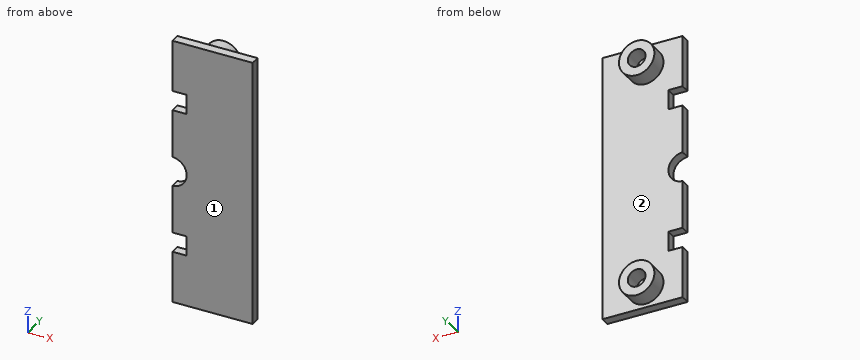
```python
from build123d import *

# Parameters (mm, degrees)
SKETCH1_W                       = 11.3
SKETCH1_H                       = 38
BASE_DEPTH                      = 1.3
SKETCH3_W                       = 2
SKETCH3_H                       = 2.8
SQUARE_NOTCH_DEPTH              = 20.864855902
SKETCH2_R                       = 2.1025
CIRCLE_DEPTH                    = 20.864855902
SKETCH4_R                       = 2.5
SKETCH4_R_2                     = 1.25
BOSSED_CYLINDER_WITH_HOLE_DEPTH = 2.4


with BuildPart() as part:
    # Sketch1 → BASE (new body)
    with BuildSketch(Plane(origin=(0, 0, 0), x_dir=(1, 0, 0), z_dir=(0, 1, 0))):
        Rectangle(SKETCH1_W, SKETCH1_H)
    extrude(amount=BASE_DEPTH)

    # Sketch3 → SQUARE NOTCH (cut, through all)
    with BuildSketch(Plane(origin=(0, 1.3, 0), x_dir=(1, 0, 0), z_dir=(0, 1, 0))):
        with Locations((-4.65, 10.3)):
            Rectangle(SKETCH3_W, SKETCH3_H)
    square_notch = extrude(amount=-SQUARE_NOTCH_DEPTH, mode=Mode.SUBTRACT)

    # SN Mirror1: SQUARE NOTCH across plane
    add(square_notch.mirror(Plane.XY), mode=Mode.SUBTRACT)

    # Sketch2 → CIRCLE (cut, through all)
    with BuildSketch(Plane(origin=(0, 1.3, 0), x_dir=(1, 0, 0), z_dir=(0, 1, 0))):
        with Locations((-5.7525, 0)):
            Circle(SKETCH2_R)
    extrude(amount=-CIRCLE_DEPTH, mode=Mode.SUBTRACT)

    # Sketch4 → BOSSED CYLINDER WITH HOLE (add)
    with BuildSketch(Plane(origin=(0, 1.3, 0), x_dir=(1, 0, 0), z_dir=(0, 1, 0))):
        with Locations(Location((-0.45, 16, 0), (0, 0, 270))):
            Circle(SKETCH4_R)
        with Locations(Location((-0.45, 16, 0), (0, 0, 270))):
            Circle(SKETCH4_R_2, mode=Mode.SUBTRACT)
    bossed_cylinder_with_hole = extrude(amount=BOSSED_CYLINDER_WITH_HOLE_DEPTH)

    # BCH Mirror2: BOSSED CYLINDER WITH HOLE across plane
    add(bossed_cylinder_with_hole.mirror(Plane.XY))


solid = part.part
```
The model under review builds one solid part; all positions refer to its coordinate system, in mm. Face numbers are marked on the shaded views. Round coordinates to 2 decimals unless told otherwise and drop trailing zeros. Order: outer loops, then holes, each group sorted by start corner. A loop starts at its lowest first (then second) coordinate and runs counter-clockwise, first axis right, second up. Notation, with made-up numbers: (69.25, -5.75) - (125.25, -5.75) arc R31 cw to (125.25, 19.25) - close; hole circle Ø1 at (-10.75, -3.75). An arc over 180 degrees is marked (long way). Answer in a Markdown table with one row per item.
(1) Take a section at A-A on z = -16. Write out the cut boundary in (x, y).
Result set:
| item | result |
|---|---|
| outline | (-5.65, 0) - (5.65, 0) - (5.65, 1.3) - (2.05, 1.3) - (2.05, 3.7) - (0.8, 3.7) - (0.8, 1.3) - (-1.7, 1.3) - (-1.7, 3.7) - (-2.95, 3.7) - (-2.95, 1.3) - (-5.65, 1.3) - close |
(2) For line 1 (X direction, y = 2.05, z = -16); line 2 (Z direction, x = -0.25, y = 2.95); line 3 (Z direction, x = -1.5, y = 2.75), list the stretches that pass through material, from the lowest coordinate up. Write a range as from..to.
Result set:
| item | result |
|---|---|
| line 1 | x = -2.95..-1.7, 0.8..2.05 |
| line 2 | z = -18.49..-17.23, -14.77..-13.51, 13.51..14.77, 17.23..18.49 |
| line 3 | z = -18.27..-16.68, -15.32..-13.73, 13.73..15.32, 16.68..18.27 |
(3) Clearance check with flat-ended pins moving along their axes: P1, Ø2, axis at x = -0.45, z = -16, coming from the -Y side; P2, Ø2, axis at x = -3, y = 3, coming from the +Z side; P3, Ø1, axis at x = -0.5, z = 0, coming from the +Y side; P4, Ø2, axis at y = 1, z = 10, coming from the -X side. State where each tip first meets the part, or that it passes through.
Result set:
| item | result |
|---|---|
| P1 | stops at y = 0 |
| P2 | stops at z = 17.96 |
| P3 | stops at y = 1.3 |
| P4 | stops at x = -3.65 |
(4) Mouldability with a two-part tool opening along Z and no side actions: class the marked faces 1 and 2 as released by +Z, released by -Z, zero draft, split by the parting line, or undercut.
Result set:
| item | result |
|---|---|
| face 1 | zero draft |
| face 2 | undercut |
(5) Take a section at C-C on x = -4. Write out the cut boundary in (y, z).
Result set:
| item | result |
|---|---|
| outline | (0, -19) - (1.3, -19) - (1.3, -11.7) - (0, -11.7) - close; (0, -8.9) - (1.3, -8.9) - (1.3, -1.16) - (0, -1.16) - close; (0, 1.16) - (1.3, 1.16) - (1.3, 8.9) - (0, 8.9) - close; (0, 11.7) - (1.3, 11.7) - (1.3, 19) - (0, 19) - close |
(6) Take a section at D-D on y = 3.25. Write out the cut boundary in (x, z).
Result set:
| item | result |
|---|---|
| outline | circle Ø5 at (-0.45, -16); circle Ø5 at (-0.45, 16); hole circle Ø2.5 at (-0.45, -16); hole circle Ø2.5 at (-0.45, 16) |
